Read the model definition and answer for the solid it produces. Units are mm, in the model's axes. A direction names the side the tool comes from. Coordinates: 2 decimals unless noted, no trailing zeros. Loops run counter-clockwise (first coordinate to the right, second up) from the corner with the lowest first, then second, coordinate; pieces in that order, holes last.
Q1. Section C-C (y = 6.75) is taken. Give the vertices of the cut face in (x, z), then the cut area to 3 significant figures.
Q2. Section A-A (x = 0) is taken. Give the vertices of the cut face in (y, z).
Q3. Section D-D (x = -3.5) is taken. Give the vertices of the cut face in (y, z).
Q4. Straight lines are drawn through the part: line 1 (X direction, y = 4, z = -13.65); line 2 (Y direction, x = 2.75, z = 0); line 3 (Y direction, x = -2, z = 7.5). For each, find the intervals that lie inside material, in ascending order.
Q5. Which of the six approach directions +Z, -Z, +X, -X, +Y, -Y give full straight-line access (tool end or side, diameter ignored) to faces 1 (the face through (7.5, 3, 0)), 2 (the face through (2, 7.3, 12)), 3 (the face through (2, 7.3, -15))?
Q6. The mould has two halves that part along Z. Classify faces 4 (the face through (-0.11, 4.08, 0.72)), 5 (the face through (0, 4, -20)), 6 (the face through (0, 0, 0)): pulls with the +Z half, pulls with the -Z half, needs draft (parallel to the pull), parting line crosses it, or undercut.
Q7. Flat-ended cylindrical pins translate along their axes: P1, Ø1, axis at x = -4, y = 12.5, coming from the -Z side; P2, Ø3, axis at x = -3, z = -9, coming from the +Y side; P3, Ø5.5, axis at y = 7.3, z = 0, coming from the -X side; P4, Ø6, axis at y = 10, z = -8.5, coming from the +X side. Find the tip coordinate at first contact, or state that the pin passes through.
Q8. Section B-B (z = -13.65) is taken. Give the vertices of the cut face in (x, y).
from build123d import *

# Parameters (mm, degrees)
CROQUIS1_R              = 3.3
SALIENTE_EXTRUIR1_DEPTH = 7.5
CORTAR_EXTRUIR1_REACH   = 24.573
CROQUIS2_R              = 2.1


with BuildPart() as part:
    # Croquis1 → Saliente-Extruir1 (new, symmetric)
    with BuildSketch(Plane(origin=(0, 0, 0), x_dir=(0, 0, -1), z_dir=(1, 0, 0))):
        with BuildLine():
            Line((-20, 0), (20, 0))
            Line((20, 0), (20, 7.3))
            Line((20, 7.3), (7.3, 7.3))
            ThreePointArc((7.3, 7.3), (0, 14.6), (-7.3, 7.3))
            Line((-7.3, 7.3), (-20, 7.3))
            Line((-20, 7.3), (-20, 0))
        make_face()
        with Locations((0, 7.3)):
            Circle(CROQUIS1_R, mode=Mode.SUBTRACT)
    extrude(amount=SALIENTE_EXTRUIR1_DEPTH, both=True)

    # Croquis2 → Cortar-Extruir1 (cut, up to next)
    with BuildSketch(Plane(origin=(0, 7.3, 0), x_dir=(1, 0, 0), z_dir=(0, 1, 0)), mode=Mode.PRIVATE) as cortar_extruir1_sk1:
        with Locations(Location((0, -13.65, 0), (0, 0, 270))):
            Circle(CROQUIS2_R)
    cortar_extruir1_tool1 = extrude(cortar_extruir1_sk1.sketch, amount=-CORTAR_EXTRUIR1_REACH, mode=Mode.PRIVATE) & part.part
    # Croquis2 → Cortar-Extruir1 (cut, up to next)
    with BuildSketch(Plane(origin=(0, 7.3, 0), x_dir=(1, 0, 0), z_dir=(0, 1, 0)), mode=Mode.PRIVATE) as cortar_extruir1_sk2:
        with Locations(Location((0, 13.65, 0), (0, 0, 270))):
            Circle(CROQUIS2_R)
    cortar_extruir1_tool2 = extrude(cortar_extruir1_sk2.sketch, amount=-CORTAR_EXTRUIR1_REACH, mode=Mode.PRIVATE) & part.part
    add(cortar_extruir1_tool1.solids().sort_by_distance((0, 7.3, 13.65))[0], mode=Mode.SUBTRACT)
    add(cortar_extruir1_tool2.solids().sort_by_distance((0, 7.3, -13.65))[0], mode=Mode.SUBTRACT)


solid = part.part
Numbers:
1. outline: (-7.5, -20) - (7.5, -20) - (7.5, -3.25) - (-7.5, -3.25) - close; (-7.5, 3.25) - (7.5, 3.25) - (7.5, 20) - (-7.5, 20) - close; hole circle Ø4.2 at (0, -13.65); hole circle Ø4.2 at (0, 13.65)
1. area: 475 mm2
2. outline: (0, -20) - (7.3, -20) - (7.3, -15.75) - (0, -15.75) - close; (0, -11.55) - (7.3, -11.55) - (7.3, -7.3) arc R7.3 ccw to (7.3, 7.3) - (7.3, 11.55) - (0, 11.55) - close; (0, 15.75) - (7.3, 15.75) - (7.3, 20) - (0, 20) - close; hole circle Ø6.6 at (7.3, 0)
3. outline: (0, -20) - (7.3, -20) - (7.3, -7.3) arc R7.3 ccw to (7.3, 7.3) - (7.3, 20) - (0, 20) - close; hole circle Ø6.6 at (7.3, 0)
4. line 1: x = -7.5 to -2.1, 2.1 to 7.5
4. line 2: y = 0 to 4, 10.6 to 14.6
4. line 3: y = 0 to 7.3
5. face 1: +Z, -Z, +X, +Y, -Y
5. face 2: +Z, +X, -X, +Y
5. face 3: -Z, +X, -X, +Y
6. face 4: undercut
6. face 5: pulls with the -Z half
6. face 6: needs draft
7. P1: stops at z = -5.59
7. P2: stops at y = 7.3
7. P3: passes through
7. P4: stops at x = 7.5
8. outline: (-7.5, 0) - (-2.1, 0) - (-2.1, 7.3) - (-7.5, 7.3) - close; (2.1, 0) - (7.5, 0) - (7.5, 7.3) - (2.1, 7.3) - close
